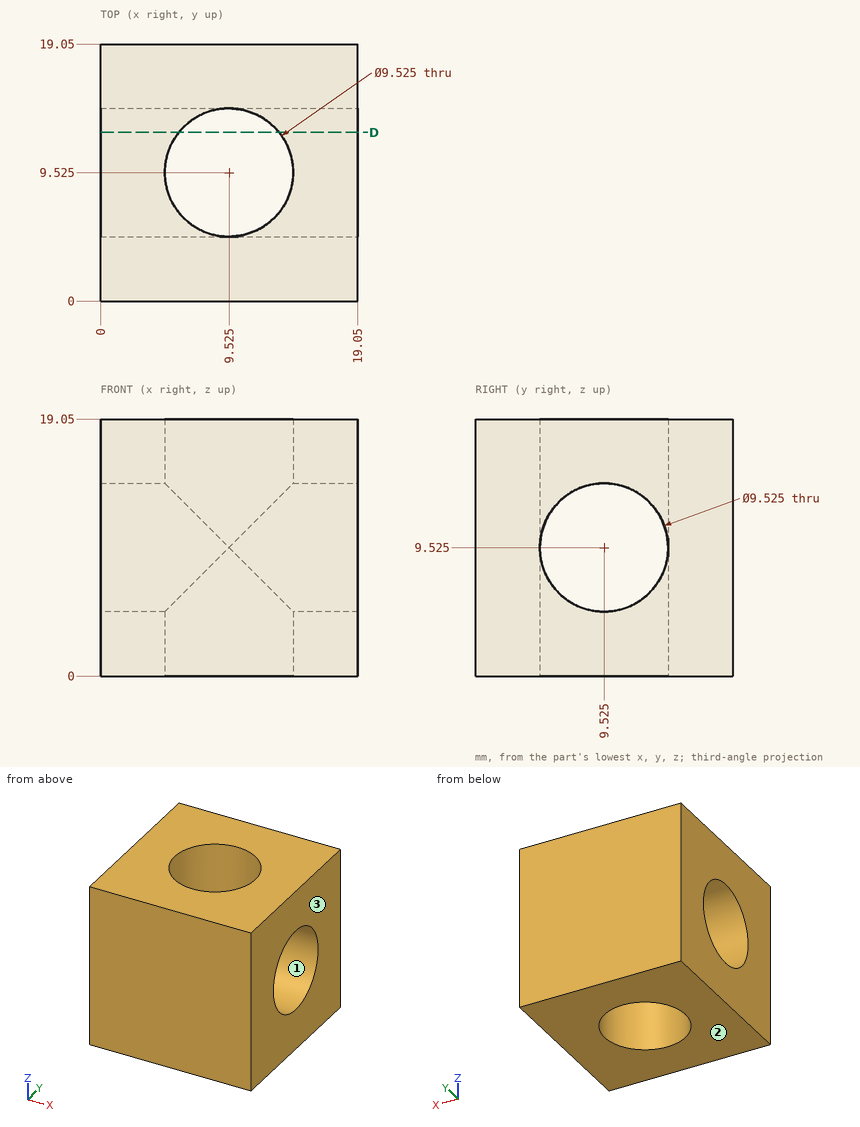
Check sheet for the drawn part. Datum: minimum x, y, z corner. Units: mm. Coordinates: 2 decimals unless noted, no trailing zeros. Order: outer loops, then holes, each group sorted by start corner. A loop starts at its lowest first (then second) coordinate and runs counter-clockwise, first axis right, second up. Notation, with made-up numbers: (89, 10.25) -> (142, 10.25) arc R15 ccw to (142, 37.25) -> close; hole circle Ø6 at (55.5, 55.25). An arc over 180 degrees is marked (long way). Use a Markdown table: item, result. Add a question column.
1. Material ranges on L1, parallel to Y at x = 10.75, z = 1; L2, parallel to Y at x = 8.5, z = 16; L3, parallel to Z at x = 17, y = 11, recorded low to high.
2. Mould release check, pull along Z, two halves, no side actions. Record for the marked faces 1, 2 and 3: pulls with the +Z half, pulls with the -Z half, needs draft (parallel to the pull), parting line crosses it, or undercut.
3. Go/stop test with a flat-tipped pin: pin 1 Ø5.5 at (y, z) = (9.525, 9.525) entering from -X. Record where the tip stops, or that it passes through.
4. Cross-section at D-D (y = 12.5). Enter the section's corners in (x, z), and give its area (3 significant figures).
Filled sheet:
| question | item | result |
|---|---|---|
| 1 | L1 | 0 to 4.92, 14.13 to 19.05 |
| 1 | L2 | 0 to 4.87, 14.18 to 19.05 |
| 1 | L3 | 0 to 5, 14.05 to 19.05 |
| 2 | face 1 | undercut |
| 2 | face 2 | pulls with the -Z half |
| 2 | face 3 | needs draft |
| 3 | pin 1 | through |
| 4 | outline | (0, 0) -> (5.81, 0) -> (5.81, 5.81) -> (0, 5.81) -> close; (0, 13.24) -> (5.81, 13.24) -> (5.81, 19.05) -> (0, 19.05) -> close; (13.24, 0) -> (19.05, 0) -> (19.05, 5.81) -> (13.24, 5.81) -> close; (13.24, 13.24) -> (19.05, 13.24) -> (19.05, 19.05) -> (13.24, 19.05) -> close |
| 4 | area | 135 mm2 |
